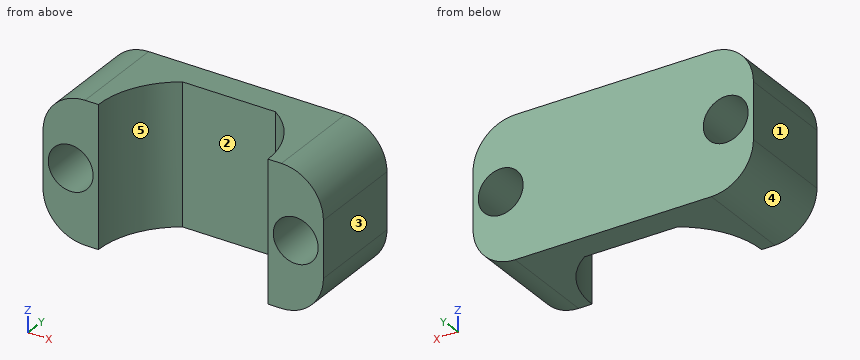
```python
from build123d import *

# Parameters (mm, degrees)
BOSS_EXTRUDE1_DEPTH = 5
SKETCH2_R           = 1.6
CUT_EXTRUDE1_DEPTH  = 14.190905958
FILLET3_R           = 3


with BuildPart() as part:
    # Sketch1 → Boss-Extrude1 (new, symmetric)
    with BuildSketch(Plane.XY):
        with BuildLine():
            Line((-10, 0), (10, 0))
            Line((10, 0), (10, -7))
            Line((10, -7), (6.05, -7))
            ThreePointArc((6.05, -7), (5.322096357, -4.135562883), (3.315, -1.966137169))
            Line((3.315, -1.966137169), (-3.315, -1.966137169))
            ThreePointArc((-3.315, -1.966137169), (-5.322096357, -4.135562883), (-6.05, -7))
            Line((-6.05, -7), (-10, -7))
            Line((-10, -7), (-10, 0))
        make_face()
    extrude(amount=BOSS_EXTRUDE1_DEPTH, both=True)

    # Sketch2 → Cut-Extrude1 (cut, through all)
    with BuildSketch(Plane.XZ.offset(7)):
        with Locations(Location((8.025, 0, 0), (0, 0, 270))):
            Circle(SKETCH2_R)
        with Locations(Location((-8.025, 0, 0), (0, 0, 270))):
            Circle(SKETCH2_R)
    extrude(amount=-CUT_EXTRUDE1_DEPTH, mode=Mode.SUBTRACT)

    # Fillet3
    fillet3_edges = [part.edges().sort_by_distance(p)[0] for p in [
        (-10, -3.5, -5),
        (10, -3.5, -5),
        (-10, -3.5, 5),
        (10, -3.5, 5),
    ]]
    fillet(fillet3_edges, radius=FILLET3_R)


solid = part.part
```
Geometry: final body of the model. Coordinates: model frame, mm. Face numbers are marked on the shaded views. A direction names the side the tool comes from. Give positions to 0.01 mm unless a question says otherwise; leave off trailing zeros. Write each loop counter-clockwise with the first axis right and the second up, starting at its lowest first coordinate (ties: lowest second). Pieces come first, ordered by that corner, then holes.
1. Reachability of the marked faces 4 and 5 from +Z, -Z, +X, -X, +Y, -Y: full face, straight path, thin tool, end or side. Return the list, or none.
2. Section query D-D, the plane y = -4.75. Return loops of the section in (x, z) (3 decimals), then the cut area to 3 significant figures.
3. Section query B-B, the plane z = 0. Return loops of the section in (x, y) (3 decimals), then the cut area to 3 significant figures.
4. Section query A-A, the plane y = -2.75. Return loops of the section in (x, z) (3 decimals).
5. Line query: probe 1 along X at (y, z) = (-4.75, 0) (3 decimals); probe 2 along X at (y, z) = (-5.25, 0) (3 decimals); probe 3 along Y at (x, z) = (2.75, 1.75). Output: solid intervals per line, ascending.
6. Pin query (flat end, axial travel): P1, Ø3.5, axis at x = 1, z = 2.5, coming from the -Y side; P2, Ø5, axis at x = 2, z = -2.5, coming from the +Y side; P3, Ø2.5, axis at x = -8.025, z = 0, coming from the -Y side. Return the tip coordinate at first contact, or that it passes through.
7. Draft query along X for the marked faces 1, 2 and 3. Return one class per face: released by +X, released by -X, zero draft, split by the parting line, or undercut.
8. Section query C-C, the plane x = -8.5. Return loops of the section in (y, z).
Computed:
1. face 4: -Z, -X, +Y, -Y
1. face 5: +Z, -Z, -Y
2. outline: (-10, -2) arc R3 ccw to (-7, -5) - (-5.612, -5) - (-5.612, 5) - (-7, 5) arc R3 ccw to (-10, 2) - close; (5.612, -5) - (7, -5) arc R3 ccw to (10, -2) - (10, 2) arc R3 ccw to (7, 5) - (5.612, 5) - close; hole circle Ø3.2 at (-8.025, 0); hole circle Ø3.2 at (8.025, 0)
2. area: 63.9 mm2
3. outline: (-10, -7) - (-9.625, -7) - (-9.625, 0) - (-10, 0) - close; (-6.425, -7) - (-6.05, -7) arc R6 cw to (-3.315, -1.966) - (3.315, -1.966) arc R6 cw to (6.05, -7) - (6.425, -7) - (6.425, 0) - (-6.425, 0) - close; (9.625, -7) - (10, -7) - (10, 0) - (9.625, 0) - close
3. area: 42.4 mm2
4. outline: (-10, -2) arc R3 ccw to (-7, -5) - (-4.285, -5) - (-4.285, 5) - (-7, 5) arc R3 ccw to (-10, 2) - close; (4.285, -5) - (7, -5) arc R3 ccw to (10, -2) - (10, 2) arc R3 ccw to (7, 5) - (4.285, 5) - close; hole circle Ø3.2 at (-8.025, 0); hole circle Ø3.2 at (8.025, 0)
5. probe 1: x = -10 to -9.625, -6.425 to -5.612, 5.612 to 6.425, 9.625 to 10
5. probe 2: x = -10 to -9.625, -6.425 to -5.789, 5.789 to 6.425, 9.625 to 10
5. probe 3: y = -1.97 to 0
6. P1: stops at y = -1.97
6. P2: stops at y = 0
6. P3: passes through
7. face 1: released by -X
7. face 2: undercut
7. face 3: released by +X
8. outline: (-7, -4.6) - (0, -4.6) - (0, -1.53) - (-7, -1.53) - close; (-7, 1.53) - (0, 1.53) - (0, 4.6) - (-7, 4.6) - close
